```python
from build123d import *

# Parameters (mm, degrees)
CROQUIS1_W              = 200
CROQUIS1_H              = 200
SALIENTE_EXTRUIR1_DEPTH = 5
CROQUIS4_R              = 3.5
CROQUIS4_R_2            = 0.9
CROQUIS4_R_3            = 3.9
CROQUIS4_R_4            = 1.4
SALIENTE_EXTRUIR3_DEPTH = 5
REDONDEO1_R             = 5
CROQUIS5_R              = 4.1
CORTAR_EXTRUIR1_DEPTH   = 5
CROQUIS7_R              = 2.5
CORTAR_EXTRUIR2_DEPTH   = 10
CROQUIS8_R              = 2.2
CROQUIS8_R_2            = 1.5875
CROQUIS8_R_3            = 1.65
CORTAR_EXTRUIR3_DEPTH   = 17


with BuildPart() as part:
    # Croquis1 → Saliente-Extruir1 (new body)
    with BuildSketch(Plane(origin=(0, 0, 0), x_dir=(0, 1, 0), z_dir=(0, 0, 1))):
        Rectangle(CROQUIS1_W, CROQUIS1_H)
    extrude(amount=SALIENTE_EXTRUIR1_DEPTH)

    # Croquis4 → Saliente-Extruir3 (add)
    # profile 1 of 14: a face of its own
    with BuildSketch(Plane.XY.offset(5)):
        with Locations((4.466366134, 32.184176934)):
            Circle(CROQUIS4_R)
        with Locations((4.466366134, 32.184176934)):
            Circle(CROQUIS4_R_2, mode=Mode.SUBTRACT)
    # profile 2 of 14: a face of its own
    with BuildSketch(Plane.XY.offset(5)):
        with Locations(Location((75.586508374, 75.364263295, 0), (0, 0, 180))):
            Circle(CROQUIS4_R)
        with Locations((75.586508374, 75.364263295)):
            Circle(CROQUIS4_R_2, mode=Mode.SUBTRACT)
    # profile 3 of 14: a face of its own
    with BuildSketch(Plane.XY.offset(5)):
        with Locations(Location((-74.976542636, 16.226296077, 0), (0, 0, 180))):
            Circle(CROQUIS4_R_3)
        with Locations((-74.976542636, 16.226296077)):
            Circle(CROQUIS4_R_4, mode=Mode.SUBTRACT)
    # profile 4 of 14: a face of its own
    with BuildSketch(Plane.XY.offset(5)):
        with Locations(Location((16.86819811, 16.226296077, 0), (0, 0, 180))):
            Circle(CROQUIS4_R_3)
        with Locations((16.86819811, 16.226296077)):
            Circle(CROQUIS4_R_4, mode=Mode.SUBTRACT)
    # profile 5 of 14: a face of its own
    with BuildSketch(Plane.XY.offset(5)):
        with Locations(Location((16.86819811, -80.452378393, 0), (0, 0, 180))):
            Circle(CROQUIS4_R_3)
        with Locations((16.86819811, -80.452378393)):
            Circle(CROQUIS4_R_4, mode=Mode.SUBTRACT)
    # profile 6 of 14: a face of its own
    with BuildSketch(Plane.XY.offset(5)):
        with Locations(Location((-74.976542636, -80.452378393, 0), (0, 0, 180))):
            Circle(CROQUIS4_R_3)
        with Locations((-74.976542636, -80.452378393)):
            Circle(CROQUIS4_R_4, mode=Mode.SUBTRACT)
    # profile 7 of 14: a face of its own
    with BuildSketch(Plane.XY.offset(5)):
        with Locations(Location((-6.408510904, 72.92167992, 0), (0, 0, 180))):
            Circle(CROQUIS4_R_3)
        with Locations((-6.408510904, 72.92167992)):
            Circle(CROQUIS4_R_4, mode=Mode.SUBTRACT)
    # profile 8 of 14: a face of its own
    with BuildSketch(Plane.XY.offset(5)):
        with Locations(Location((-6.408510904, 34.92167992, 0), (0, 0, 180))):
            Circle(CROQUIS4_R_3)
        with Locations((-6.408510904, 34.92167992)):
            Circle(CROQUIS4_R_4, mode=Mode.SUBTRACT)
    # profile 9 of 14: a face of its own
    with BuildSketch(Plane.XY.offset(5)):
        with Locations(Location((-74.408510904, 34.92167992, 0), (0, 0, 180))):
            Circle(CROQUIS4_R_3)
        with Locations((-74.408510904, 34.92167992)):
            Circle(CROQUIS4_R_4, mode=Mode.SUBTRACT)
    # profile 10 of 14: a face of its own
    with BuildSketch(Plane.XY.offset(5)):
        with Locations(Location((4.466366134, 75.364263295, 0), (0, 0, 180))):
            Circle(CROQUIS4_R)
        with Locations((4.466366134, 75.364263295)):
            Circle(CROQUIS4_R_2, mode=Mode.SUBTRACT)
    # profile 11 of 14: a face of its own
    with BuildSketch(Plane.XY.offset(5)):
        with Locations(Location((75.586508374, 32.184176934, 0), (0, 0, 180))):
            Circle(CROQUIS4_R)
        with Locations((75.586508374, 32.184176934)):
            Circle(CROQUIS4_R_2, mode=Mode.SUBTRACT)
    # profile 12 of 14: a face of its own
    with BuildSketch(Plane.XY.offset(5)):
        with Locations(Location((-74.408510904, 72.92167992, 0), (0, 0, 180))):
            Circle(CROQUIS4_R_3)
        with Locations((-74.408510904, 72.92167992)):
            Circle(CROQUIS4_R_4, mode=Mode.SUBTRACT)
    # profile 13 of 14: a face of its own
    with BuildSketch(Plane.XY.offset(5)):
        with BuildLine():
            Line((32.455622465, 6.933114513), (36.757832016, 6.933114513))
            Line((36.757832016, 6.933114513), (36.757832016, 2.449848629))
            ThreePointArc((36.757832016, 2.449848629), (41.041030118, 10.865935643), (32.455622465, 6.933114513))
        make_face()
    # profile 14 of 14: a face of its own
    with BuildSketch(Plane.XY.offset(5)):
        with BuildLine():
            Line((29.611177214, 6.933114513), (25.086009497, 6.933114513))
            Line((25.086009497, 6.933114513), (25.086009497, 2.424526913))
            ThreePointArc((25.086009497, 2.424526913), (21.104360825, 10.946016112), (29.611177214, 6.933114513))
        make_face()
    extrude(amount=SALIENTE_EXTRUIR3_DEPTH)

    # Redondeo1
    redondeo1_edges = [part.edges().sort_by_distance(p)[0] for p in [
        (100, 100, 2.5),
        (100, -100, 2.5),
        (-100, -100, 2.5),
        (-100, 100, 2.5),
    ]]
    fillet(redondeo1_edges, radius=REDONDEO1_R)

    # Croquis5 → Cortar-Extruir1 (cut)
    with BuildSketch(Plane(origin=(0, 0, 5), x_dir=(0, -1, 0), z_dir=(0, 0, 1))):
        with Locations(Location((-92.5, -92.5, 0), (0, 0, 90))):
            Circle(CROQUIS5_R)
        with Locations(Location((92.5, -92.5, 0), (0, 0, 90))):
            Circle(CROQUIS5_R)
        with Locations(Location((92.5, 92.5, 0), (0, 0, 90))):
            Circle(CROQUIS5_R)
        with Locations(Location((-92.5, 92.5, 0), (0, 0, 90))):
            Circle(CROQUIS5_R)
    extrude(amount=-CORTAR_EXTRUIR1_DEPTH, mode=Mode.SUBTRACT)

    # Croquis7 → Cortar-Extruir2 (cut)
    with BuildSketch(Plane(origin=(0, 0, 0), x_dir=(1, 0, 0), z_dir=(0, 0, -1))):
        with Locations(Location((77.341864461, -18.038506913, 0), (0, 0, 180))):
            Circle(CROQUIS7_R)
        with Locations(Location((54.891864461, 67.961493087, 0), (0, 0, 180))):
            Circle(CROQUIS7_R)
    extrude(amount=-CORTAR_EXTRUIR2_DEPTH, mode=Mode.SUBTRACT)

    # Croquis8 → Cortar-Extruir3 (cut)
    with BuildSketch(Plane.XY.offset(10)):
        with Locations(Location((37.433399839, 7.403999224, 0), (0, 0, 252.116878215))):
            Circle(CROQUIS8_R)
        with Locations(Location((24.633399839, 7.403999224, 0), (0, 0, 347.64087537))):
            Circle(CROQUIS8_R)
        with Locations((-74.976542636, -80.452378393)):
            Circle(CROQUIS8_R_2)
        with Locations((16.86819811, -80.452378393)):
            Circle(CROQUIS8_R_2)
        with Locations((16.86819811, 16.226296077)):
            Circle(CROQUIS8_R_2)
        with Locations((-74.976542636, 16.226296077)):
            Circle(CROQUIS8_R_2)
        with Locations((-6.408510904, 34.92167992)):
            Circle(CROQUIS8_R_3)
        with Locations((-6.408510904, 72.92167992)):
            Circle(CROQUIS8_R_3)
        with Locations((-74.408510904, 72.92167992)):
            Circle(CROQUIS8_R_3)
        with Locations((-74.408510904, 34.92167992)):
            Circle(CROQUIS8_R_3)
    extrude(amount=-CORTAR_EXTRUIR3_DEPTH, mode=Mode.SUBTRACT)


solid = part.part
```
The listing builds one solid part. Answer for the finished solid, in the listing's coordinates (mm). A direction names the side the tool comes from. Give positions to 0.01 mm unless a question says otherwise; leave off trailing zeros. Order: outer loops, then holes, each group sorted by start corner. A loop starts at its lowest first (then second) coordinate and runs counter-clockwise, first axis right, second up.
Item 1: Given pin 1 Ø2.5 at (y, z) = (4, 8.5) entering from -X; pin 2 Ø12 at (x, y) = (45.5, -42.5) entering from +Z; pin 3 Ø4 at (x, z) = (20, 9) entering from +Y, each flat-ended and moving along its own axis, determine where each tip first touches the part or whether it passes through.
From the geometry:
pin 1: stops at x = 20.12
pin 2: stops at z = 5
pin 3: stops at y = 19.96
Item 2: Which of the six approach directions +Z, -Z, +X, -X, +Y, -Y give full straight-line access (tool end or side, diameter ignored) to faces 1 (the face through (39.346, 8.491, 5.07)), 2 (the face through (41.16, 10.74, 7.46))?
From the geometry:
face 1: +Z, -Z
face 2: +Z
Item 3: Find the intervals of material crossed by probe 1 along Y at (x, z) = (-74.5, 4.5); probe 2 along Z at (x, y) = (-57, 1); probe 3 along X at (y, z) = (9, 9.5), in increasing order.
From the geometry:
probe 1: y = -100 to -81.97, -78.94 to 14.71, 17.74 to 33.27, 36.57 to 71.27, 74.57 to 100
probe 2: z = 0 to 5
probe 3: x = 19.89 to 23.12, 26.15 to 29.37, 32.69 to 35.92, 38.95 to 42.17
Item 4: The part is cut by section A-A, the plane x = 92.5. Give the vertices of the cut face in (y, z).
From the geometry:
outline: (-100, 0) - (-96.6, 0) - (-96.6, 5) - (-100, 5) - close; (-88.4, 0) - (88.4, 0) - (88.4, 5) - (-88.4, 5) - close; (96.6, 0) - (100, 0) - (100, 5) - (96.6, 5) - close
Item 5: The part is cut by section C-C, the plane x = -61. Give the vertices of the cut face in (y, z).
From the geometry:
outline: (-100, 0) - (100, 0) - (100, 5) - (-100, 5) - close
Item 6: For a pull along Y with two mould halves and no side action, classify faces 3 (the face through (1, -100, 2)), 4 (the face through (3.7, 76.1, 10)), 5 (the face through (-5.901, 69.055, 7.465)) as pulls with the +Y half, pulls with the -Y half, needs draft (parallel to the pull), parting line crosses it, or undercut.
From the geometry:
face 3: pulls with the -Y half
face 4: needs draft
face 5: undercut
